Input: part model. Units: mm. Frame: model coordinates. Face numbers are marked on the shaded views. A direction names the side the tool comes from. Give positions to 0.01 mm unless a question says otherwise; leave off trailing zeros. Write each loop counter-clockwise with the first axis right and the second up, starting at its lowest first coordinate (ties: lowest second). Pieces come first, ordered by that corner, then holes. Notation, with made-up numbers: (-16, -12.75) - (43, -12.75) arc R17 cw to (43, 18.25) - close; hole circle Ø9 at (15.25, 1.5). An arc over 180 degrees is marked (long way). Answer as CSV lines item,"result".
```python
from build123d import *

# Parameters (mm, degrees)
BOSS_EXTRUDE1_DEPTH            = 6.35
M5_CLEARANCE_HOLE2_D           = 5.5
M5_CLEARANCE_HOLE2_DEPTH       = 10.1
M5_CLEARANCE_HOLE2_CSINK_D     = 5.55
M5_CLEARANCE_HOLE2_CSINK_ANGLE = 90
M5_CLEARANCE_HOLE2_TIP         = 1.652366702


with BuildPart() as part:
    # Sketch1 → Boss-Extrude1 (new body)
    with BuildSketch(Plane(origin=(0, 0, 0), x_dir=(1, 0, 0), z_dir=(0, 1, 0))):
        Polygon((10.749371316, 22.5), (0.749371316, 22.5), (0.749371316, 4.762050808), (3.498742631, 0), (0.749371316, -4.762050808), (0.749371316, -22.5), (10.749371316, -22.5), align=None)
    extrude(amount=BOSS_EXTRUDE1_DEPTH)

    # M5 Clearance Hole2
    with Locations(Plane(origin=(0, 6.35, 0), x_dir=(1, 0, 0), z_dir=(0, 1, 0))):
        with Locations((5.749371316, 15), (5.749371316, -15)):
            CounterSinkHole(M5_CLEARANCE_HOLE2_D / 2, M5_CLEARANCE_HOLE2_CSINK_D / 2, depth=M5_CLEARANCE_HOLE2_DEPTH, counter_sink_angle=M5_CLEARANCE_HOLE2_CSINK_ANGLE)
            with Locations((0, 0, -(M5_CLEARANCE_HOLE2_DEPTH + M5_CLEARANCE_HOLE2_TIP / 2))):  # 118° drill point
                Cone(0, M5_CLEARANCE_HOLE2_D / 2, M5_CLEARANCE_HOLE2_TIP, mode=Mode.SUBTRACT)


solid = part.part
```
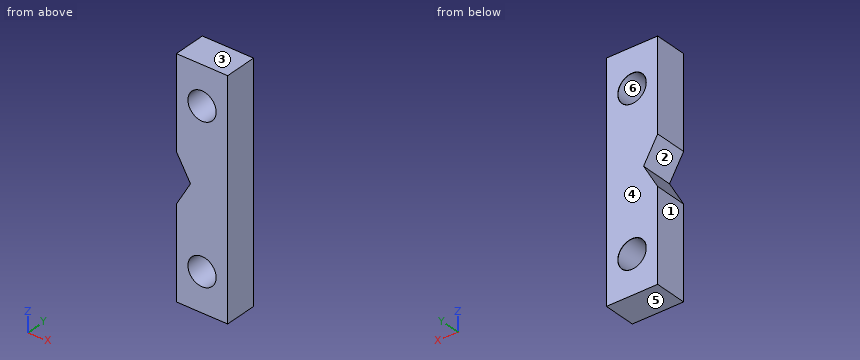
Item 1: Cut plane B-B on z = -15. Return the cut outline in (x, y) (3 decimals).
The answers:
outline,"(0.749, 0) - (2.999, 0) - (2.999, 6.325) - (2.974, 6.35) - (0.749, 6.35) - close; (8.499, 0) - (10.749, 0) - (10.749, 6.35) - (8.524, 6.35) - (8.499, 6.325) - close"
Item 2: Mould query, pull axis Z, two halves, no side actions, for the marked faces 3, 4, 5 and 6. Classes: +Z half, -Z half, draft (parallel to the pull), parting line (faces both ways), or undercut.
The answers:
face 3,"+Z half"
face 4,"draft"
face 5,"-Z half"
face 6,"undercut"
Item 3: Cut plane A-A on y = 3.25. Return the cut outline in (x, z), plus the area to 3 significant figures.
The answers:
outline,"(0.75, -22.5) - (10.75, -22.5) - (10.75, 22.5) - (0.75, 22.5) - (0.75, 4.76) - (3.5, 0) - (0.75, -4.76) - close; hole circle Ø5.5 at (5.75, -15); hole circle Ø5.5 at (5.75, 15)"
area,"389 mm²"
Item 4: Cut plane C-C on x = 2.25. Return the cut outline in (y, z).
The answers:
outline,"(0, -22.5) - (6.35, -22.5) - (6.35, -2.16) - (0, -2.16) - close; (0, 2.16) - (6.35, 2.16) - (6.35, 22.5) - (0, 22.5) - close"
Item 5: Ray query, line 1 (X direction, y = 5, z = 15); line 2 (Z direction, x = 4.75, y = 3.75); line 3 (Z direction, x = 8.25, y = 4). Return the intervals inside material, ascending. Write a range as from..to.
The answers:
line 1,"0.75..3, 8.5..10.75"
line 2,"-22.5..-17.56, -12.44..12.44, 17.56..22.5"
line 3,"-22.5..-16.14, -13.86..13.86, 16.14..22.5"
Item 6: Reachability of the marked faces 1 and 2 from +Z, -Z, +X, -X, +Y, -Y: full face, straight path, thin tool, end or side. Return the list, or none.
The answers:
face 1,"+Z, -Z, -X, +Y, -Y"
face 2,"-X, +Y, -Y"
Item 7: Cut plane D-D on x = 7.75. Count the separate pieces of the cut face and the enclosed holes in it, plus the area to 3 significant figures.
The answers:
separate pieces,"3"
enclosed holes,"0"
area,"238 mm²"
